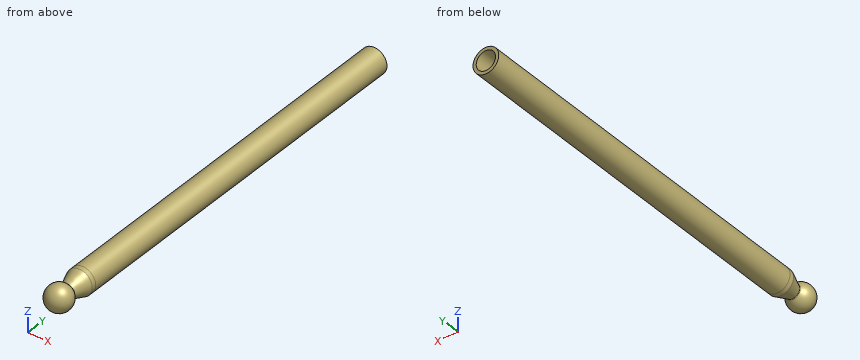
```python
from build123d import *

# Parameters (mm, degrees)
SKETCH1_R           = 40
EXTRUDE1_DEPTH      = 1200
SKETCH2_R           = 30
CUT_EXTRUDE1_DEPTH  = 800
SKETCH_1_R          = 10
CUT_EXTRUDE_1_DEPTH = 35.6


# Read off the part's stored shape, not the designer's step: 连接重组1
with BuildPart() as part:
    # Sketch1 → Extrude1 (new body)
    with BuildSketch(Plane(origin=(0, 0, 0), x_dir=(1, 0, 0), z_dir=(0, 1, 0))):
        with Locations(Location((0, 0, 0), (0, 0, 270))):
            Circle(SKETCH1_R)
    extrude(amount=-EXTRUDE1_DEPTH)

    # Sketch2 → Cut-Extrude1 (cut)
    with BuildSketch(Plane(origin=(0, 0, 0), x_dir=(1, 0, 0), z_dir=(0, 1, 0))):
        with Locations(Location((0, 0, 0), (0, 0, 270))):
            Circle(SKETCH2_R)
    extrude(amount=-CUT_EXTRUDE1_DEPTH, mode=Mode.SUBTRACT)

    # 草图1 → 切除-拉伸1 (cut)
    with BuildSketch(Plane.XZ.offset(1200)):
        with Locations(Location((0, 0, 0), (0, 0, 270))):
            Circle(SKETCH_1_R)
    extrude(amount=-CUT_EXTRUDE_1_DEPTH, mode=Mode.SUBTRACT)

    # 连接重组1 outline → 连接重组1 (revolve)
    with BuildSketch(Plane.XY):
        with BuildLine():
            ThreePointArc((0, -1337.73332), (38.089361999, -1309.948085758), (23.262631735, -1265.193345126))
            ThreePointArc((23.262631735, -1265.193345126), (22.516451416, -1264.161768918), (22.543988515, -1262.888907458))
            Line((22.543988515, -1262.888907458), (39.999998202, -1214.399991661))
            Line((39.999998202, -1214.399991661), (40, -1200))
            Line((40, -1200), (10, -1200))
            Line((10, -1200), (10, -1164.4))
            Line((10, -1164.4), (0, -1164.4))
            Line((0, -1164.4), (0, -1337.73332))
        make_face()
    revolve(axis=Axis((0, 0, 0), (0, 1, 0)))


solid = part.part
```
Input: part model. Units: mm. Frame: model coordinates. Coordinates: 2 decimals unless noted, no trailing zeros. Order: outer loops, then holes, each group sorted by start corner. A loop starts at its lowest first (then second) coordinate and runs counter-clockwise, first axis right, second up. Notation, with made-up numbers: (66.5, -40) - (115.5, -40) arc R14 cw to (115.5, -23) - close; hole circle Ø8 at (13.25, 47.5). An arc over 180 degrees is marked (long way). Put each result on its own line as item: value.
1. Cut plane A-A on y = -88.5. Return the cut outline in (x, z), then the cut area to 3 significant figures.
Report:
outline: circle Ø80 at (0, 0); hole circle Ø60 at (0, 0)
area: 2,200 mm2
2. Contact query for flat-ended pins moving along their axis: pin 1 Ø1 at (y, z) = (-309, 30.5) entering from +X; pin 2 Ø1.5 at (x, z) = (8.5, 16) entering from +Y; pin 3 Ø3 at (y, z) = (-670.5, 19) entering from +X. Output: stop coordinate, or through.
Report:
pin 1: stops at x = 26.46
pin 2: stops at y = -800
pin 3: stops at x = 35.97
3. Line query: line 1 along X through (y, z) = (-587, 0); line 2 along Z through (x, y) = (2, -425.5); line 3 along Z through (x, y) = (-10, -349). Output: solid intervals per line, ascending.
Report:
line 1: x = -40 to -30, 30 to 40
line 2: z = -39.95 to -29.93, 29.93 to 39.95
line 3: z = -38.73 to -28.28, 28.28 to 38.73
4. Cut plane C-C on y = -1044. Return the cut outline in (x, z), then the cut area to 3 significant figures.
Report:
outline: circle Ø80 at (0, 0)
area: 5,030 mm2
5. Cut plane B-B on x = 0. Return the cut outline in (y, z).
Report:
outline: (-1265.19, -23.26) arc R2 cw to (-1262.89, -22.54) - (-1214.4, -40) - (0, -40) - (0, -30) - (-800, -30) - (-800, 30) - (0, 30) - (0, 40) - (-1214.4, 40) - (-1262.89, 22.54) arc R2 cw to (-1265.19, 23.26) arc R40 ccw (long way) to start
